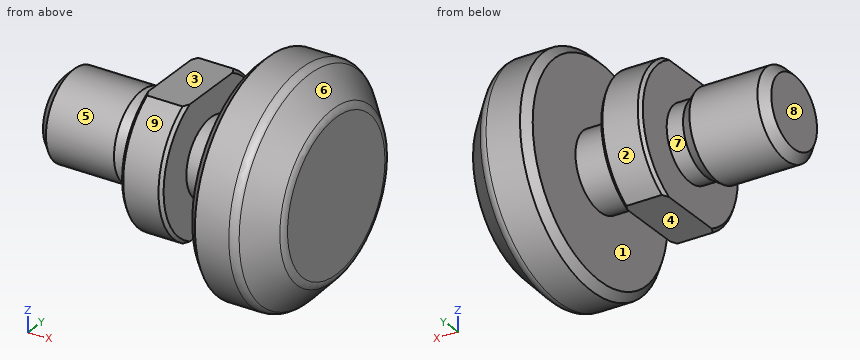
Autodesk Inventor part; units mm, degrees
ref_plane "side_1_XY" through (9.5, 0, 0) normal (-1, 0, 0) x (0, 0, -1)
ref_plane "side_1_YZ" through (9.5, 0, 0) normal (0, 0, -1) x (0, -1, 0)
ref_plane "side_1_ZX" through (9.5, 0, 0) normal (0, -1, 0) x (-1, 0, 0)
sketch "Skizze_1" plane through (0, 0, 0) normal (0, 0, 1) x (1, 0, 0)
  line L0 (24.75, 0) -> (0, 0)
  line L1 (0, 0) -> (0, 3.233)
  line L2 (0, 3.233) -> (0.767, 4)
  line L3 (0.767, 4) -> (7, 4)
  line L4 (7, 4) -> (8, 3.35)
  line L5 (8, 3.35) -> (9.5, 3.35)
  line L6 (9.5, 3.35) -> (9.5, 6.7172)
  line L7 (9.5, 6.7172) -> (9.7828, 7)
  line L8 (9.7828, 7) -> (13.0172, 7)
  line L9 (13.0172, 7) -> (13.3, 6.7172)
  line L10 (13.3, 6.7172) -> (13.3, 3.5)
  line L11 (13.3, 3.5) -> (17.75, 3.5)
  line L12 (17.75, 3.5) -> (17.75, 9.5429)
  line L13 (17.75, 9.5429) -> (18.4571, 10.25)
  line L14 (18.4571, 10.25) -> (21.5622, 10.25)
  arc A0 (22.297, 9.9283) -> (21.5622, 10.25) centre (21.5622, 9.25) ccw
  line L15 (22.297, 9.9283) -> (24.4848, 7.5581)
  arc A1 (24.75, 6.8798) -> (24.4848, 7.5581) centre (23.75, 6.8798) ccw
  line L16 (24.75, 6.8798) -> (24.75, 0)
  line L17 (24.75, 0) -> (0, 0)
revolve "Revolution1" add sketch "Skizze_1" angle 360 about axis through (24.75, 0, 0) along (1, 0, 0)
thread "Thread1"
sketch "Skizze_2" plane through (0, 0, 0) normal (0, 1, 0) x (-1, 0, 0)
  line L0 (-6, 6) -> (-6, 14)
  line L1 (-6, 14) -> (-14, 14)
  line L2 (-14, 14) -> (-14, 6)
  line L3 (-14, 6) -> (-6, 6)
extrude "Extrusion1" cut sketch "Skizze_2" along normal mid plane 10
sketch "Skizze_3" plane through (0, 0, 0) normal (0, 1, 0) x (-1, 0, 0)
  line L0 (-6, -14) -> (-6, -6)
  line L1 (-6, -6) -> (-14, -6)
  line L2 (-14, -6) -> (-14, -14)
  line L3 (-14, -14) -> (-6, -14)
extrude "Extrusion2" cut sketch "Skizze_3" along normal mid plane 10
ref_plane "side_1_XY" through (9.5, 0, 0) normal (-1, 0, 0) x (0, 0, -1)
ref_plane "side_1_YZ" through (9.5, 0, 0) normal (0, 0, -1) x (0, -1, 0)
ref_plane "side_1_ZX" through (9.5, 0, 0) normal (0, -1, 0) x (-1, 0, 0)
ref_plane "side_2_XY" through (14.6, 0, 0) normal (1, 0, 0) x (0, 0, -1)
ref_plane "side_2_YZ" through (14.6, 0, 0) normal (0, 0, -1) x (0, 1, 0)
ref_plane "side_2_ZX" through (14.6, 0, 0) normal (0, 1, 0) x (1, 0, 0)
properties part number "MayTec 1.67.42E3M8_Slot roller E3"
Input: part model. Units: mm. Frame: model coordinates. Face numbers are marked on the shaded views. A direction names the side the tool comes from. Round coordinates to 2 decimals unless told otherwise and drop trailing zeros. Order: outer loops, then holes, each group sorted by start corner. A loop starts at its lowest first (then second) coordinate and runs counter-clockwise, first axis right, second up. Notation, with made-up numbers: (-34, 79.5) - (-14, 79.5) arc R26 ccw to (-14, 109.5) - close; hole circle Ø2 at (-21, -28.5). An arc over 180 degrees is marked (long way). Answer as a JSON object with one key per item and string values. Group by question number.
(1) Pin query (flat end, axial travel): P1, Ø6, axis at y = -3, z = -7.5, coming from the -X side; P2, Ø3, axis at x = 11, y = -1, coming from the +Z side; P3, Ø1, axis at x = 22, y = 2.5, coming from the +Z side. Return the tip coordinate at first contact, or that it passes through.
(2) Draft query along X for the marked faces 6, 7, 8 and 9. Return one class per face: released by +X, released by -X, zero draft, split by the parting line, or undercut.
(3) Material intervals for probe 1 along X at (y, z) = (-4.5, -4.75); probe 2 along X at (y, z) = (3.75, -0.75); probe 3 along Z at (x, y) = (13, -5.75), sorted ascending. Write a range as from..to.
(4) Cut plane C-C (x = 16.25). Return loops of the section in (y, z).
(5) Reachability of the marked faces 1, 2, 3, 4 and 5 from +Z, -Z, +X, -X, +Y, -Y: full face, straight path, thin tool, end or side. Return the list, or none.
Here are the results:
{
 "1": {"P1": "stops at x = 9.5", "P2": "stops at z = 6", "P3": "stops at z = 10.02"},
 "2": {"face 6": "released by +X", "face 7": "undercut", "face 8": "released by -X", "face 9": "zero draft"},
 "3": {"probe 1": "x = 9.5..13.3, 17.75..24.75", "probe 2": "x = 0.59..7.27, 9.5..13.3, 17.75..24.75", "probe 3": "z = -3.99..3.99"},
 "4": {"outline": "circle Ø7 at (0, 0)"},
 "5": {"face 1": "none", "face 2": "-X, +Y", "face 3": "+Z, -X, +Y, -Y", "face 4": "-Z, -X, +Y, -Y", "face 5": "-X"}
}
